```python
from build123d import *

# Parameters (mm, degrees)
BOSS_EXTRUDE1_START = -7.320002
SKETCH1_R           = 1.38
SKETCH1_R_2         = 1.6
BOSS_EXTRUDE1_DEPTH = 7.520002
BOSS_EXTRUDE2_START = -8.920002
SKETCH1_3_R         = 1.6
BOSS_EXTRUDE2_DEPTH = 1.6
BOSS_EXTRUDE3_START = 0.2
SKETCH1_4_R         = 1.6
SKETCH1_4_R_2       = 1.38
SKETCH1_4_R_3       = 3.995
SKETCH1_4_R_4       = 1.995
BOSS_EXTRUDE3_DEPTH = 1.5


with BuildPart() as part:
    # Sketch1 → Boss-Extrude1 (new body)
    with BuildSketch(Plane.ZY.offset(18.486711134).offset(BOSS_EXTRUDE1_START)):
        with BuildLine():
            ThreePointArc((-12.870344381, -12.708128144), (-11.997005912, -9.823687124), (-9.670344381, -7.908128144))
            Line((-9.670344381, -7.908128144), (-12.470344381, -7.908128144))
            ThreePointArc((-12.470344381, -7.908128144), (-16.005878287, -9.372594238), (-17.470344381, -12.908128144))
            Line((-17.470344381, -12.908128144), (-17.470344381, -30.276049303))
            ThreePointArc((-17.470344381, -30.276049303), (-16.005878287, -33.811583208), (-12.470344381, -35.276049303))
            Line((-12.470344381, -35.276049303), (9.844655619, -35.276049303))
            ThreePointArc((9.844655619, -35.276049303), (11.612422572, -34.543816256), (12.344655619, -32.776049303))
            Line((12.344655619, -32.776049303), (12.344655619, -30.076049303))
            Line((12.344655619, -30.076049303), (-7.670344381, -30.076049303))
            ThreePointArc((-7.670344381, -30.076049303), (-11.347299643, -28.553004565), (-12.870344381, -24.876049303))
            Line((-12.870344381, -24.876049303), (-12.870344381, -12.708128144))
        make_face()
        with Locations((-15.070344381, -18.823128144)):
            Circle(SKETCH1_R, mode=Mode.SUBTRACT)
        with Locations((8.844655619, -32.676049303)):
            Circle(SKETCH1_R_2, mode=Mode.SUBTRACT)
    extrude(amount=BOSS_EXTRUDE1_DEPTH)

    # Sketch1<3> → Boss-Extrude2 (add)
    with BuildSketch(Plane.ZY.offset(18.486711134).offset(BOSS_EXTRUDE2_START)):
        with BuildLine():
            ThreePointArc((-12.870344381, -12.708128144), (-11.997005912, -9.823687124), (-9.670344381, -7.908128144))
            Line((-9.670344381, -7.908128144), (-12.470344381, -7.908128144))
            ThreePointArc((-12.470344381, -7.908128144), (-16.005878287, -9.372594238), (-17.470344381, -12.908128144))
            Line((-17.470344381, -12.908128144), (-17.470344381, -16.123128144))
            Line((-17.470344381, -16.123128144), (-13.753187094, -16.123128144))
            Line((-13.753187094, -16.123128144), (-12.870344381, -15.240285432))
            Line((-12.870344381, -15.240285432), (-12.870344381, -12.708128144))
        make_face()
        with BuildLine():
            Line((12.344655619, -32.776049303), (12.344655619, -30.076049303))
            Line((12.344655619, -30.076049303), (-7.670344381, -30.076049303))
            ThreePointArc((-7.670344381, -30.076049303), (-11.347299643, -28.553004565), (-12.870344381, -24.876049303))
            Line((-12.870344381, -24.876049303), (-12.870344381, -22.405970857))
            Line((-12.870344381, -22.405970857), (-13.753187094, -21.523128144))
            Line((-13.753187094, -21.523128144), (-17.470344381, -21.523128144))
            Line((-17.470344381, -21.523128144), (-17.470344381, -30.276049303))
            ThreePointArc((-17.470344381, -30.276049303), (-16.005878287, -33.811583208), (-12.470344381, -35.276049303))
            Line((-12.470344381, -35.276049303), (9.844655619, -35.276049303))
            ThreePointArc((9.844655619, -35.276049303), (11.612422572, -34.543816256), (12.344655619, -32.776049303))
        make_face()
        with Locations((8.844655619, -32.676049303)):
            Circle(SKETCH1_3_R, mode=Mode.SUBTRACT)
    extrude(amount=BOSS_EXTRUDE2_DEPTH)

    # Sketch1<4> → Boss-Extrude3 (add)
    with BuildSketch(Plane.ZY.offset(18.486711134).offset(BOSS_EXTRUDE3_START)):
        with BuildLine():
            ThreePointArc((-12.870344381, -24.876049303), (-11.347299643, -28.553004565), (-7.670344381, -30.076049303))
            Line((-7.670344381, -30.076049303), (12.344655619, -30.076049303))
            Line((12.344655619, -30.076049303), (12.344655619, -32.776049303))
            ThreePointArc((12.344655619, -32.776049303), (11.612422572, -34.543816256), (9.844655619, -35.276049303))
            Line((9.844655619, -35.276049303), (-12.470344381, -35.276049303))
            ThreePointArc((-12.470344381, -35.276049303), (-16.005878287, -33.811583208), (-17.470344381, -30.276049303))
            Line((-17.470344381, -30.276049303), (-17.470344381, -21.523128144))
            Line((-17.470344381, -21.523128144), (-13.753187094, -21.523128144))
            Line((-13.753187094, -21.523128144), (-12.870344381, -22.405970857))
            Line((-12.870344381, -22.405970857), (-12.870344381, -24.876049303))
        make_face()
        with Locations((8.844655619, -32.676049303)):
            Circle(SKETCH1_4_R, mode=Mode.SUBTRACT)
        with BuildLine():
            ThreePointArc((-9.670344381, -7.908128144), (-11.997005912, -9.823687124), (-12.870344381, -12.708128144))
            Line((-12.870344381, -12.708128144), (-12.870344381, -15.240285432))
            Line((-12.870344381, -15.240285432), (-13.753187094, -16.123128144))
            Line((-13.753187094, -16.123128144), (-17.470344381, -16.123128144))
            Line((-17.470344381, -16.123128144), (-17.470344381, -12.908128144))
            ThreePointArc((-17.470344381, -12.908128144), (-16.005878287, -9.372594238), (-12.470344381, -7.908128144))
            Line((-12.470344381, -7.908128144), (-9.670344381, -7.908128144))
        make_face()
        Polygon((-12.870344381, -22.405970857), (-12.870344381, -15.240285432), (-13.753187094, -16.123128144), (-17.470344381, -16.123128144), (-17.470344381, -21.523128144), (-13.753187094, -21.523128144), align=None)
        with Locations((-15.070344381, -18.823128144)):
            Circle(SKETCH1_4_R_2, mode=Mode.SUBTRACT)
        with BuildLine():
            Line((12.344655619, -29.376049303), (12.344655619, -8.208128144))
            Line((12.344655619, -8.208128144), (-7.670344381, -8.208128144))
            ThreePointArc((-7.670344381, -8.208128144), (-10.852324897, -9.526147629), (-12.170344381, -12.708128144))
            Line((-12.170344381, -12.708128144), (-12.170344381, -24.876049303))
            ThreePointArc((-12.170344381, -24.876049303), (-10.852324897, -28.058029818), (-7.670344381, -29.376049303))
            Line((-7.670344381, -29.376049303), (12.344655619, -29.376049303))
        make_face()
        with Locations((-1.750344381, -18.823128144)):
            Circle(SKETCH1_4_R_3, mode=Mode.SUBTRACT)
        with Locations((9.499655619, -18.823128144)):
            Circle(SKETCH1_4_R_4, mode=Mode.SUBTRACT)
        with BuildLine():
            Line((12.344655619, -7.908128144), (-9.670344381, -7.908128144))
            ThreePointArc((-9.670344381, -7.908128144), (-11.997005912, -9.823687124), (-12.870344381, -12.708128144))
            Line((-12.870344381, -12.708128144), (-12.870344381, -15.240285432))
            Line((-12.870344381, -15.240285432), (-12.870344381, -22.405970857))
            Line((-12.870344381, -22.405970857), (-12.870344381, -24.876049303))
            ThreePointArc((-12.870344381, -24.876049303), (-11.347299643, -28.553004565), (-7.670344381, -30.076049303))
            Line((-7.670344381, -30.076049303), (12.344655619, -30.076049303))
            Line((12.344655619, -30.076049303), (12.344655619, -29.376049303))
            Line((12.344655619, -29.376049303), (-7.670344381, -29.376049303))
            ThreePointArc((-7.670344381, -29.376049303), (-10.852324897, -28.058029818), (-12.170344381, -24.876049303))
            Line((-12.170344381, -24.876049303), (-12.170344381, -12.708128144))
            ThreePointArc((-12.170344381, -12.708128144), (-10.852324897, -9.526147629), (-7.670344381, -8.208128144))
            Line((-7.670344381, -8.208128144), (12.344655619, -8.208128144))
            Line((12.344655619, -8.208128144), (12.344655619, -7.908128144))
        make_face()
    extrude(amount=BOSS_EXTRUDE3_DEPTH)


solid = part.part
```
Verification items for the finished model (mm, model axes). A direction names the side the tool comes from. Round coordinates to 2 decimals unless told otherwise and drop trailing zeros. Loops run counter-clockwise (first coordinate to the right, second up) from the corner with the lowest first, then second, coordinate; pieces in that order, holes last. Notation, with made-up numbers: (16, 47.25) -> (66, 47.25) arc R25 cw to (66, 78.25) -> close; hole circle Ø3 at (20, 46.5). An arc over 180 degrees is marked (long way). Answer as a JSON object with one key per item and string values.
Q1. Scan lines: line 1 (Y direction, x = -17.5, z = -6.5); line 2 (X direction, y = -11.75, z = 3); line 3 (Z direction, x = -12.75, y = -22.25). Record each from-to range of solid material in increasing order. Write a range as from..to.
Data:
{"line 1": "y = -35.28..-30.08", "line 2": "x = -20.19..-18.69", "line 3": "z = -17.47..-12.87"}
Q2. Section check C-C (z = 3). Record the boundary of the cut face in (x, y).
Data:
{"outline": "(-20.19, -35.28) -> (-9.57, -35.28) -> (-9.57, -30.08) -> (-18.69, -30.08) -> (-18.69, -7.91) -> (-20.19, -7.91) -> close"}
Q3. Draft check along Z on faces 1 (the flat face through (-15, -21, -17.47)), 2 (the cylindrical face through (-14.1, -28.6, -11.3)), 3 (the cylindrical face through (-14.8, -31.09, 8.64)). Enter one of: pulls with the +Z half, pulls with the -Z half, needs draft (parallel to the pull), parting line crosses it, or undercut.
Data:
{"face 1": "pulls with the -Z half", "face 2": "pulls with the +Z half", "face 3": "undercut"}
Q4. Section check D-D (x = -12.5). Record the boundary of the cut face in (y, z), then the cut area to 3 significant figures.
Data:
{"outline": "(-35.28, -12.47) arc R5 ccw to (-30.28, -17.47) -> (-12.91, -17.47) arc R5 ccw to (-7.91, -12.47) -> (-7.91, -9.67) arc R5.2 cw to (-12.71, -12.87) -> (-24.88, -12.87) arc R5.2 cw to (-30.08, -7.67) -> (-30.08, 12.34) -> (-32.78, 12.34) arc R2.5 ccw to (-35.28, 9.84) -> close; hole circle Ø3.2 at (-32.68, 8.84); hole circle Ø2.76 at (-18.82, -15.07)", "area": "241 mm2"}
Q5. Section check B-B (y = -19.5). Record the boundary of the cut face in (x, z), then the cut area to 3 significant figures.
Data:
{"outline": "(-20.19, -17.47) -> (-11.17, -17.47) -> (-11.17, -16.27) -> (-20.19, -16.27) -> close; (-20.19, -13.87) -> (-11.17, -13.87) -> (-11.17, -12.87) -> (-18.69, -12.87) -> (-18.69, -5.69) -> (-20.19, -5.69) -> close; (-20.19, 2.19) -> (-18.69, 2.19) -> (-18.69, 7.62) -> (-20.19, 7.62) -> close; (-20.19, 11.38) -> (-18.69, 11.38) -> (-18.69, 12.34) -> (-20.19, 12.34) -> close", "area": "40.2 mm2"}
Q6. Access from +Z, -Z, +X, -X, +Y, -Y to the whole of each face (thin tool, end or side, straight path). Record for faces 4 (the cylindrical face through (-15.614, -17.455, -15.25)), 5 (the flat face through (-10, -16.123, -16)), 6 (the flat face through (-14, -19, -12.87)).
Data:
{"face 4": "+X, -X", "face 5": "+Z, -Z, +X", "face 6": "+Z, +X"}
Q7. Section check A-A (z = 8.25). Record the boundary of the cut face in (x, y), then the cut area to 3 significant figures.
Data:
{"outline": "(-20.19, -35.28) -> (-9.57, -35.28) -> (-9.57, -34.16) -> (-20.19, -34.16) -> close; (-20.19, -31.19) -> (-9.57, -31.19) -> (-9.57, -30.08) -> (-18.69, -30.08) -> (-18.69, -20.38) -> (-20.19, -20.38) -> close; (-20.19, -17.27) -> (-18.69, -17.27) -> (-18.69, -7.91) -> (-20.19, -7.91) -> close", "area": "52.3 mm2"}
Q8. Go/stop test with flat-tipped pins: P1, Ø0.8, axis at x = -10, z = -15.5, coming from the -Y side; P2, Ø5, axis at x = -15, z = -3.5, coming from the +Y side; P3, Ø3.5, axis at y = -18.5, z = -16, coming from the +X side. Record where each tip stops, or that it passes through.
Data:
{"P1": "stops at y = -34.53", "P2": "stops at y = -30.08", "P3": "stops at x = -11.17"}
